from build123d import *

# Parameters (mm, degrees)
F0_R      = 200
F1_DEPTH  = 1800
F2_W      = 130
F2_H      = 170
F3_DEPTH  = 500
F4_W      = 50
F4_H      = 50
F5_DEPTH  = 500
F8_W      = 50
F8_H      = 50
F9_DEPTH  = 500
F11_W     = 50
F11_H     = 50
F12_DEPTH = 500
F13_R     = 20


with BuildPart() as f1:
    # F0 (on Top) → F1 (new body)
    with BuildSketch(Plane.XY):
        Circle(F0_R)
    extrude(amount=-F1_DEPTH)

    # F2 (on Front) → F3 (cut, symmetric)
    with BuildSketch(Plane.XZ):
        with Locations((0, -1215)):
            Rectangle(F2_W, F2_H)
    extrude(amount=F3_DEPTH, both=True, mode=Mode.SUBTRACT)

    # F4 (on Front) → F5 (cut, symmetric)
    with BuildSketch(Plane.XZ):
        with Locations((0, -725)):
            Rectangle(F4_W, F4_H)
    extrude(amount=F5_DEPTH, both=True, mode=Mode.SUBTRACT)

    # F8 (on face) → F9 (cut, symmetric)
    with BuildSketch(Plane(origin=(0, 0, 0), x_dir=(-0.965926, -0.258819, 0), z_dir=(-0.258819, 0.965926, 0))):
        with Locations((-75, -425)):
            Rectangle(F8_W, F8_H)
    extrude(amount=F9_DEPTH, both=True, mode=Mode.SUBTRACT)

    # F11 (on face) → F12 (cut, symmetric)
    with BuildSketch(Plane(origin=(0, 0, 0), x_dir=(-0.866025, 0.5, 0), z_dir=(0.5, 0.866025, 0))):
        with Locations((-117.285978, -365)):
            Rectangle(F11_W, F11_H)
    extrude(amount=F12_DEPTH, both=True, mode=Mode.SUBTRACT)

    # F13
    f13_edges = [f1.edges().sort_by_distance(p)[0] for p in [
        (-200, 0, 0),
    ]]
    fillet(f13_edges, radius=F13_R)


solid = f1.part
The model under review builds one solid part; all positions refer to its coordinate system, in mm. A direction names the side the tool comes from. Coordinates: 2 decimals unless noted, no trailing zeros. Loops run counter-clockwise (first coordinate to the right, second up) from the corner with the lowest first, then second, coordinate; pieces in that order, holes last. Notation, with made-up numbers: (-15.75, -22.75) -> (20.25, -22.75) arc R33 ccw to (20.25, 11.25) -> close; hole circle Ø9 at (-18, 1). An arc over 180 degrees is marked (long way). Use a Markdown table: item, result. Add a question column.
1. Add section C-C on z = -882.5. Write out the cut boundary in (x, y).
2. Add section A-A on z = -1266. Write out the cut boundary in (x, y).
3. Clearance check with flat-ended pins moving along their axes: pin 1 Ø1.5 at (y, z) = (96.5, -299.5) entering from -X; pin 2 Ø2 at (x, z) = (-120.5, -421.5) entering from -Y; pin 3 Ø1.5 at (y, z) = (99.5, -656) entering from +X. State where each tip first meets the part, or that it passes through.
4. Add section D-D on y = -157.5. Give the number of separate pieces and of enclosed holes in the cut face, plus the area to 3 significant figures.
5. Machinability: for faces 1 (the face through (65, -3, -1216)), 2 (the face through (-3, 3, 0)), 3 (the face through (72, 22, -400)), which of the approach directions +Z, -Z, +X, -X, +Y, -Y give a long, thin tool a straight path to every point of the face, cutting with its end or side? Answer none if there is none.
6. To check wall thickness, follow line 1 (Z direction, x = -0.5, y = -131); line 2 (Z direction, x = -39.5, y = 127); line 3 (X direction, y = 6.5, z = -177.5). State the ranges of each line that lie inside material, in increasing order.
7. Draft analysis for pull direction Y (two halves, no side actions). For faces 4 (the face through (124.207, -69.439, -365.35)), 5 (the face through (0, -3, -750)), state which applies: pulls with the +Y half, pulls with the -Y half, needs draft (parallel to the pull), parting line crosses it, or undercut.
8. Add section B-B on y = 0. Write out the cut boundary in (x, z).
Returned:
| question | item | result |
|---|---|---|
| 1 | outline | circle Ø400 at (0, 0) |
| 2 | outline | (-65, -189.14) -> (-65, 189.14) arc R200 ccw to start; (65, -189.14) arc R200 ccw to (65, 189.14) -> close |
| 3 | pin 1 | stops at x = -175.59 |
| 3 | pin 2 | stops at y = -160.37 |
| 3 | pin 3 | stops at x = 173.92 |
| 4 | separate pieces | 1 |
| 4 | enclosed holes | 3 |
| 4 | area | 415,000 mm² |
| 5 | face 1 | +Y, -Y |
| 5 | face 2 | +Z, +X, -X, +Y, -Y |
| 5 | face 3 | none |
| 6 | line 1 | z = -1800 to -1300, -1130 to -750, -700 to 0 |
| 6 | line 2 | z = -1800 to -1300, -1130 to 0 |
| 6 | line 3 | x = -199.89 to 199.89 |
| 7 | face 4 | undercut |
| 7 | face 5 | needs draft |
| 8 | outline | (-200, -1800) -> (200, -1800) -> (200, -20) arc R20 ccw to (180, 0) -> (-180, 0) arc R20 ccw to (-200, -20) -> close; hole (-65, -1300) -> (65, -1300) -> (65, -1130) -> (-65, -1130) -> close; hole (-25, -750) -> (25, -750) -> (25, -700) -> (-25, -700) -> close; hole (51.76, -450) -> (103.53, -450) -> (103.53, -400) -> (51.76, -400) -> close; hole (106.56, -390) -> (164.3, -390) -> (164.3, -340) -> (106.56, -340) -> close |
